from build123d import *

# Parameters (mm, degrees)
SALIENTE_EXTRUIR1_DEPTH = 10
CORTAR_EXTRUIR1_DEPTH   = 2
SALIENTE_EXTRUIR2_DEPTH = 2
CROQUIS5_R              = 1.4
CROQUIS5_R_2            = 2.5
CORTAR_EXTRUIR2_DEPTH   = 5
CROQUIS6_R              = 15
CORTAR_EXTRUIR3_DEPTH   = 1
CROQUIS7_R              = 11
CROQUIS7_R_2            = 4
SALIENTE_EXTRUIR3_DEPTH = 3


with BuildPart() as part:
    # Croquis2 → Saliente-Extruir1 (new body)
    with BuildSketch(Plane.XY):
        Polygon((-16, 21), (16, 21), (21, 15), (21, -15), (16, -21), (-16, -21), (-21, -15), (-21, 15), align=None)
    extrude(amount=SALIENTE_EXTRUIR1_DEPTH)

    # Croquis3 → Cortar-Extruir1 (cut)
    with BuildSketch(Plane.XY.offset(10)):
        Polygon((-14, 20), (14, 20), (20, 13.004934109), (20, -13.004934109), (14, -20), (-14, -20), (-20, -13.004934109), (-20, 13.004934109), align=None)
    extrude(amount=-CORTAR_EXTRUIR1_DEPTH, mode=Mode.SUBTRACT)

    # Croquis4 → Saliente-Extruir2 (add)
    with BuildSketch(Plane.XY.offset(10)):
        Polygon((-16, -21), (-14, -20), (-20, -13.004934109), (-21, -15), align=None)
        Polygon((-20, 13.004934109), (-14, 20), (-16, 21), (-21, 15), (-21, 12.992008233), align=None)
        Polygon((16, 21), (21, 15), (20, 13.004934109), (14, 20), align=None)
        Polygon((16, -21), (21, -15), (20, -13.004934109), (14, -20), align=None)
    extrude(amount=SALIENTE_EXTRUIR2_DEPTH)

    # Croquis5 → Cortar-Extruir2 (cut)
    with BuildSketch(Plane(origin=(0, 0, 0), x_dir=(-1, 0, 0), z_dir=(0, 0, -1))):
        with Locations((15.5, 15.5)):
            Circle(CROQUIS5_R)
        with Locations((-15.5, 15.5)):
            Circle(CROQUIS5_R)
        with Locations((15.5, -15.5)):
            Circle(CROQUIS5_R)
        with Locations((-15.5, -15.5)):
            Circle(CROQUIS5_R)
        Circle(CROQUIS5_R_2)
    extrude(amount=-CORTAR_EXTRUIR2_DEPTH, mode=Mode.SUBTRACT)

    # Croquis6 → Cortar-Extruir3 (cut)
    with BuildSketch(Plane(origin=(0, 0, 0), x_dir=(-1, 0, 0), z_dir=(0, 0, -1))):
        Circle(CROQUIS6_R)
    extrude(amount=-CORTAR_EXTRUIR3_DEPTH, mode=Mode.SUBTRACT)

    # Croquis7 → Saliente-Extruir3 (add)
    with BuildSketch(Plane(origin=(0, 0, 1), x_dir=(-1, 0, 0), z_dir=(0, 0, -1))):
        Circle(CROQUIS7_R)
        Circle(CROQUIS7_R_2, mode=Mode.SUBTRACT)
    extrude(amount=SALIENTE_EXTRUIR3_DEPTH)


solid = part.part
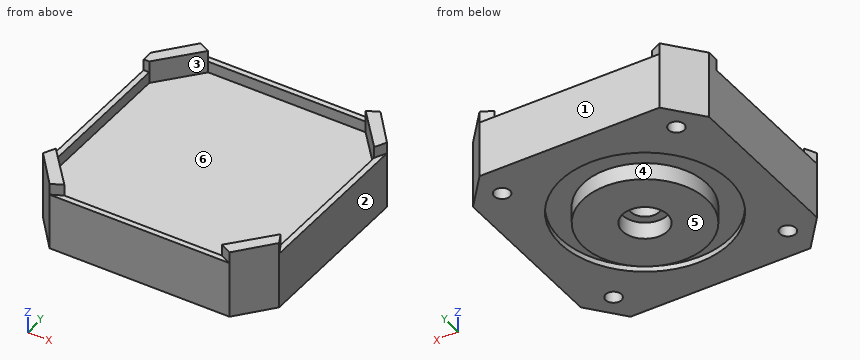
Read the model definition and answer for the solid it produces. Units are mm, in the model's axes. Face numbers are marked on the shaded views. A direction names the side the tool comes from. Coordinates: 2 decimals unless noted, no trailing zeros. Loops run counter-clockwise (first coordinate to the right, second up) from the corner with the lowest first, then second, coordinate; pieces in that order, holes last.
Q1. The part is cut by section B-B on y = -12. Write down the section's boundary in (x, z).
Q2. The part is cut by section D-D on x = 0. Write down the section's boundary in (y, z), and give its area (3 significant figures).
Q3. Consider probe 1 along Y at (x, z) = (0, 0.8); probe 2 along Y at (x, z) = (2, 9); probe 3 along Y at (x, z) = (0, 2.6). Determine where each line is inside the solid, lowest interval first.
Q4. The part is cut by section C-C on z = 4.25. Write down the section's boundary in (x, y).
Q5. The mould has two halves that part along Y. Classify the marked faces 1, 2 and 3: +Y half, -Y half, draft (parallel to the pull), parting line (faces both ways), or undercut.
Q6. Each of these flat-tipped pins is pushed along its axis until it touches: pin 1 Ø1.5 at (x, y) = (0, 1) entering from -Z; pin 2 Ø0.5 at (x, y) = (-2, 20.5) entering from +Z; pin 3 Ø2.5 at (x, y) = (-1.5, -0.5) entering from -Z. Where does it stop, or does it pass through?
Q7. Which of the six approach directions +Z, -Z, +X, -X, +Y, -Y give full straight-line access (tool end or side, diameter ignored) to the marked faces 4, 5 and 6?
Q8. The part is cut by section A-A on z = 10.5. Write down the section's boundary in (x, y), and give its area (3 significant figures).
Results below:
1. outline: (-21, 0) - (-9, 0) - (-9, 1) - (9, 1) - (9, 0) - (21, 0) - (21, 10) - (20, 10) - (20, 8) - (-20, 8) - (-20, 10) - (-21, 10) - close
2. outline: (-21, 0) - (-15, 0) - (-15, 1) - (-11, 1) - (-11, -2) - (-4, -2) - (-4, 1) - (-2.5, 1) - (-2.5, 5) - (2.5, 5) - (2.5, 1) - (4, 1) - (4, -2) - (11, -2) - (11, 1) - (15, 1) - (15, 0) - (21, 0) - (21, 10) - (20, 10) - (20, 8) - (-20, 8) - (-20, 10) - (-21, 10) - close
2. area: 332 mm2
3. probe 1: y = -21 to -15, -11 to -4, 4 to 11, 15 to 21
3. probe 2: y = -21 to -20, 20 to 21
3. probe 3: y = -21 to -2.5, 2.5 to 21
4. outline: (-21, -15) - (-16, -21) - (16, -21) - (21, -15) - (21, 15) - (16, 21) - (-16, 21) - (-21, 15) - close; hole circle Ø2.8 at (-15.5, -15.5); hole circle Ø2.8 at (-15.5, 15.5); hole circle Ø5 at (0, 0); hole circle Ø2.8 at (15.5, -15.5); hole circle Ø2.8 at (15.5, 15.5)
5. face 1: +Y half
5. face 2: draft
5. face 3: undercut
6. pin 1: stops at z = 5
6. pin 2: stops at z = 10
6. pin 3: stops at z = 1
7. face 4: -Z
7. face 5: -Z, +X, -X, +Y, -Y
7. face 6: +Z
8. outline: (-21, -15) - (-16, -21) - (-14, -20) - (-20, -13) - close; (-21, 12.99) - (-20, 13) - (-14, 20) - (-16, 21) - (-21, 15) - close; (14, -20) - (16, -21) - (21, -15) - (20, -13) - close; (14, 20) - (20, 13) - (21, 15) - (16, 21) - close
8. area: 72.9 mm2
